The listing builds one solid part. Answer for the finished solid, in the listing's coordinates (mm). Face numbers are marked on the shaded views. A direction names the side the tool comes from. Coordinates: 2 decimals unless noted, no trailing zeros. Order: outer loops, then holes, each group sorted by start corner. A loop starts at its lowest first (then second) coordinate and runs counter-clockwise, first axis right, second up. Notation, with made-up numbers: (40.5, 2.25) -> (57.5, 2.25) arc R31 ccw to (57.5, 39.25) -> close; hole circle Ø9 at (-24, -30). An arc over 180 degrees is marked (long way). Answer in a Markdown table with one row per item.
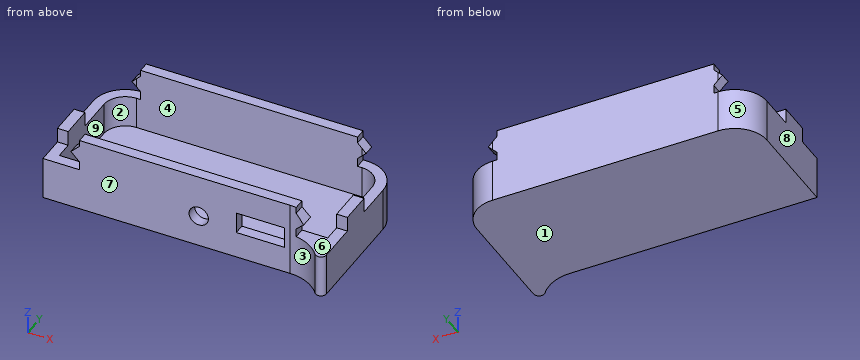
```python
from build123d import *

# Parameters (mm, degrees)
PAD018_DEPTH    = 14
POCKET026_DEPTH = 12
FILLET004_R     = 1
POCKET029_DEPTH = 27.344146
SKETCH088_R     = 1.8
SKETCH088_W     = 9
SKETCH088_H     = 4
POCKET030_DEPTH = 2
SKETCH090_W     = 2
SKETCH090_H     = 6
PAD020_DEPTH    = 2.8


with BuildPart() as part:
    # Sketch079 → Pad018 (new body)
    with BuildSketch(Plane.XY):
        with BuildLine():
            Line((40, 105.4), (82, 105.4))
            ThreePointArc((88, 99.4), (86.242641, 103.642641), (82, 105.4))
            Line((88, 99.4), (88, 73.4))
            ThreePointArc((88, 73.4), (85.656854, 79.056854), (80, 81.4))
            Line((80, 81.4), (34, 81.4))
            Line((34, 81.4), (34, 99.4))
            ThreePointArc((40, 105.4), (35.757359, 103.642641), (34, 99.4))
        make_face()
    extrude(amount=PAD018_DEPTH)

    # Sketch076 → Pocket026 (cut)
    with BuildSketch(Plane.XY.offset(2)):
        with BuildLine():
            Line((40, 103.4), (82, 103.4))
            ThreePointArc((86, 99.4), (84.828427, 102.228427), (82, 103.4))
            Line((86, 99.4), (86, 83.4))
            Line((86, 83.4), (36, 83.4))
            Line((36, 83.4), (36, 99.4))
            ThreePointArc((40, 103.4), (37.171573, 102.228427), (36, 99.4))
        make_face()
    extrude(amount=POCKET026_DEPTH, mode=Mode.SUBTRACT)

    # Fillet004
    fillet004_edges = [part.edges().sort_by_distance(p)[0] for p in [
        (88, 73.4, 7),
    ]]
    fillet(fillet004_edges, radius=FILLET004_R)

    # Sketch087 (on DatumPlane) → Pocket029 (cut, through all)
    with BuildSketch(Plane(origin=(0, 105.4, 0), x_dir=(-1, 0, 0), z_dir=(0, 1, 0))):
        Polygon((-88, 14), (-81.2, 14), (-81.2, 12.8), (-82.8, 11.2), (-81.2, 9.6), (-81.2, 8), (-88, 8), align=None)
        Polygon((-40.8, 14), (-34, 14), (-34, 8), (-40.8, 8), (-40.8, 9.6), (-39.2, 11.2), (-40.8, 12.8), align=None)
    extrude(amount=-POCKET029_DEPTH, mode=Mode.SUBTRACT)

    # Sketch088 (on DatumPlane) → Pocket030 (cut)
    with BuildSketch(Plane.XZ.offset(-81.4)):
        with Locations((63, 6)):
            Circle(SKETCH088_R)
        with Locations((74.5, 7)):
            Rectangle(SKETCH088_W, SKETCH088_H)
    extrude(amount=-POCKET030_DEPTH, mode=Mode.SUBTRACT)

    # Sketch090 (on DatumPlane) → Pad020 (join)
    with BuildSketch(Plane.XY.offset(8)):
        with Locations((35, 89.6)):
            Rectangle(SKETCH090_W, SKETCH090_H)
        with Locations((87, 89.6)):
            Rectangle(SKETCH090_W, SKETCH090_H)
    extrude(amount=PAD020_DEPTH)


solid = part.part
```
(1) Which of the six approach directions +Z, -Z, +X, -X, +Y, -Y give full straight-line access (tool end or side, diameter ignored) to the marked faces 5, 6, 7, 8 and 9?
Check values:
| item | result |
|---|---|
| face 5 | +Z, -Z, -X, +Y |
| face 6 | +X, -Y |
| face 7 | +Z, -Z, -X, -Y |
| face 8 | +Z, -Z, -X, +Y, -Y |
| face 9 | +Z |
(2) Find the intervals of material crossed by line 1 along Y through (x, z) = (54, 8.5); line 2 along X through (y, z) = (92.5, 10.5); line 3 along Z through (x, y) = (63, 82.6), in increasing order. Write a range as from..to.
Check values:
| item | result |
|---|---|
| line 1 | 81.4..83.4, 103.4..105.4 |
| line 2 | 34..36, 86..88 |
| line 3 | 0..4.2, 7.8..14 |
(3) A cutting plane is placed at B-B, the plane z = 6. Determine the outline of the cut face in (x, y).
Check values:
| item | result |
|---|---|
| outline | (34, 81.4) -> (61.2, 81.4) -> (61.2, 83.4) -> (36, 83.4) -> (36, 99.4) arc R4 cw to (40, 103.4) -> (82, 103.4) arc R4 cw to (86, 99.4) -> (86, 83.4) -> (79, 83.4) -> (79, 81.4) -> (80, 81.4) arc R8 cw to (86.22, 78.43) arc R1 ccw to (88, 79.06) -> (88, 99.4) arc R6 ccw to (82, 105.4) -> (40, 105.4) arc R6 ccw to (34, 99.4) -> close; (64.8, 81.4) -> (70, 81.4) -> (70, 83.4) -> (64.8, 83.4) -> close |
(4) A cutting plane is placed at D-D, the plane x = 84. Determine the outline of the cut face in (y, z).
Check values:
| item | result |
|---|---|
| outline | (80.33, 0) -> (105.06, 0) -> (105.06, 8) -> (102.86, 8) -> (102.86, 2) -> (83.4, 2) -> (83.4, 8) -> (80.33, 8) -> close |
(5) For a pull along Y with two mould halves and no side action, classify the marked faces 1, 2, 3 and 4 as released by +Y, released by -Y, zero draft, split by the parting line, or undercut.
Check values:
| item | result |
|---|---|
| face 1 | zero draft |
| face 2 | undercut |
| face 3 | released by -Y |
| face 4 | undercut |
(6) A cutting plane is placed at A-A, the plane x = 63. Determine the outline of the cut face in (y, z).
Check values:
| item | result |
|---|---|
| outline | (81.4, 0) -> (105.4, 0) -> (105.4, 14) -> (103.4, 14) -> (103.4, 2) -> (83.4, 2) -> (83.4, 4.2) -> (81.4, 4.2) -> close; (81.4, 7.8) -> (83.4, 7.8) -> (83.4, 14) -> (81.4, 14) -> close |
(7) A cutting plane is placed at C-C, the plane y = 91.5. Determine the outline of the cut face in (x, z).
Check values:
| item | result |
|---|---|
| outline | (34, 0) -> (88, 0) -> (88, 10.8) -> (86, 10.8) -> (86, 2) -> (36, 2) -> (36, 10.8) -> (34, 10.8) -> close |
(8) Flat-ended cylindrical pins translate along their axes: pin 1 (1.6 mm diameter, centred on x = 35.5, y = 84.5, fed in from +Z); pin 2 (4 mm diameter, centred on x = 56, z = 6.5, fed in from -Y); pin 3 (0.6 mm diameter, centred on x = 86.5, y = 88.5, fed in from +Z). Find the tip coordinate at first contact, or state that the pin passes through.
Check values:
| item | result |
|---|---|
| pin 1 | z = 8 |
| pin 2 | y = 81.4 |
| pin 3 | z = 10.8 |
